Input: part model. Units: mm. Frame: model coordinates. A direction names the side the tool comes from. Coordinates: 2 decimals unless noted, no trailing zeros. Order: outer loops, then holes, each group sorted by start corner. A loop starts at its lowest first (then second) coordinate and runs counter-clockwise, first axis right, second up. Notation, with made-up numbers: (85.5, 15.25) - (93.5, 15.25) arc R13 cw to (93.5, 39.25) - close; hole circle Ø8 at (-19.75, 88.5). An arc over 180 degrees is marked (long way). Use a Markdown table: item, result. Add a question column.
from build123d import *

# Parameters (mm, degrees)
SKETCH_2_R             = 5
EXTRUDE_1_DEPTH        = 0.8
SKETCH_3_W             = 55
SKETCH_3_H             = 2
EXTRUDE_2_DEPTH        = 22
SKETCH_4_R             = 3
EXTRUDE_3_DEPTH        = 2
PATTERN_LINEAR_1_COUNT = 2
PATTERN_LINEAR_1_PITCH = 98
SKETCH_5_R             = 1.6
SKETCH_5_R_2           = 9.5
CUT_EXTRUDE_1_DEPTH    = 2


with BuildPart() as part:
    # 草图2 → 凸台-拉伸1 (new, symmetric)
    with BuildSketch(Plane(origin=(0, 0, 0), x_dir=(1, 0, 0), z_dir=(0, 1, 0))):
        Polygon((-127.5, 75), (-127.5, -75), (-93.5, -75), (-93.5, -48), (-11, -48), (-11, -75), (11, -75), (11, -48), (93.5, -48), (93.5, -75), (127.5, -75), (127.5, 75), (93.5, 75), (93.5, 48), (11, 48), (11, 75), (-11, 75), (-11, 48), (-93.5, 48), (-93.5, 75), align=None)
        with Locations(Location((0, 0, 0), (0, 0, 270))):
            Circle(SKETCH_2_R, mode=Mode.SUBTRACT)
    extrude(amount=EXTRUDE_1_DEPTH, both=True)

    # 草图3 → 凸台-拉伸2 (add)
    with BuildSketch(Plane(origin=(0, 0.8, 0), x_dir=(1, 0, 0), z_dir=(0, 1, 0))):
        with Locations((-44, -47)):
            Rectangle(SKETCH_3_W, SKETCH_3_H)
        with Locations((44, -47)):
            Rectangle(SKETCH_3_W, SKETCH_3_H)
        with Locations((44, 47)):
            Rectangle(SKETCH_3_W, SKETCH_3_H)
        with Locations((-44, 47)):
            Rectangle(SKETCH_3_W, SKETCH_3_H)
    extrude(amount=EXTRUDE_2_DEPTH)

    # 草图4 → 凸台-拉伸3 (add)
    with BuildSketch(Plane.XY.offset(48)):
        with Locations((55.5, 11.8)):
            Circle(SKETCH_4_R)
        with Locations(Location((-55.5, 11.8, 0), (0, 0, 180))):
            Circle(SKETCH_4_R)
    extrude_3 = extrude(amount=EXTRUDE_3_DEPTH)

    # 阵列(线性)1: 凸台-拉伸3 ×2
    with Locations(*[(0, 0, -i * PATTERN_LINEAR_1_PITCH) for i in range(1, PATTERN_LINEAR_1_COUNT)]):
        add(extrude_3)

    # 草图5 → 切除-拉伸1 (cut)
    with BuildSketch(Plane.XZ.offset(0.8)):
        with Locations(Location((-55.5, 0, 0), (0, 0, 270))):
            Circle(SKETCH_5_R)
        with Locations(Location((0, 56.5, 0), (0, 0, 270))):
            Circle(SKETCH_5_R)
        with Locations(Location((7, 70, 0), (0, 0, 270))):
            Circle(SKETCH_5_R)
        with Locations(Location((-7, 70, 0), (0, 0, 270))):
            Circle(SKETCH_5_R)
        with Locations(Location((99, 50, 0), (0, 0, 270))):
            Circle(SKETCH_5_R)
        with Locations(Location((-81.5, -42.5, 0), (0, 0, 270))):
            Circle(SKETCH_5_R)
        with Locations(Location((-50.5, -42.5, 0), (0, 0, 270))):
            Circle(SKETCH_5_R)
        with Locations(Location((-99, -50, 0), (0, 0, 270))):
            Circle(SKETCH_5_R)
        with Locations(Location((-97, 0, 0), (0, 0, 270))):
            Circle(SKETCH_5_R_2)
        with Locations(Location((-121.5, -7, 0), (0, 0, 270))):
            Circle(SKETCH_5_R)
        with Locations(Location((55.5, 0, 0), (0, 0, 90))):
            Circle(SKETCH_5_R)
        with Locations(Location((81.5, -42.5, 0), (0, 0, 90))):
            Circle(SKETCH_5_R)
        with Locations(Location((50.5, -42.5, 0), (0, 0, 90))):
            Circle(SKETCH_5_R)
        with Locations(Location((99, -50, 0), (0, 0, 90))):
            Circle(SKETCH_5_R)
        with Locations(Location((121.5, -7, 0), (0, 0, 90))):
            Circle(SKETCH_5_R)
        with Locations(Location((97, 0, 0), (0, 0, 270))):
            Circle(SKETCH_5_R_2)
        with Locations(Location((7, -70, 0), (0, 0, 90))):
            Circle(SKETCH_5_R)
        with Locations(Location((-7, -70, 0), (0, 0, 90))):
            Circle(SKETCH_5_R)
        with Locations(Location((0, -56.5, 0), (0, 0, 90))):
            Circle(SKETCH_5_R)
        with Locations(Location((50.5, 42.5, 0), (0, 0, 270))):
            Circle(SKETCH_5_R)
        with Locations(Location((81.5, 42.5, 0), (0, 0, 270))):
            Circle(SKETCH_5_R)
        with Locations(Location((121.5, 7, 0), (0, 0, 270))):
            Circle(SKETCH_5_R)
        with Locations(Location((-50.5, 42.5, 0), (0, 0, 90))):
            Circle(SKETCH_5_R)
        with Locations(Location((-121.5, 7, 0), (0, 0, 90))):
            Circle(SKETCH_5_R)
        with Locations(Location((-81.5, 42.5, 0), (0, 0, 90))):
            Circle(SKETCH_5_R)
        with Locations(Location((-99, 50, 0), (0, 0, 90))):
            Circle(SKETCH_5_R)
        with Locations(Location((-79.5, 19, 0), (0, 0, 270))):
            Circle(SKETCH_5_R)
        with Locations(Location((-41.5, 19, 0), (0, 0, 270))):
            Circle(SKETCH_5_R)
        with Locations(Location((-41.5, -19, 0), (0, 0, 90))):
            Circle(SKETCH_5_R)
        with Locations(Location((-79.5, -19, 0), (0, 0, 270))):
            Circle(SKETCH_5_R)
        with Locations(Location((41.5, 19, 0), (0, 0, 90))):
            Circle(SKETCH_5_R)
        with Locations(Location((79.5, 19, 0), (0, 0, 90))):
            Circle(SKETCH_5_R)
        with Locations(Location((41.5, -19, 0), (0, 0, 270))):
            Circle(SKETCH_5_R)
        with Locations(Location((79.5, -19, 0), (0, 0, 270))):
            Circle(SKETCH_5_R)
    extrude(amount=-CUT_EXTRUDE_1_DEPTH, mode=Mode.SUBTRACT)


solid = part.part
1) Cut plane A-A (y = 4.5). Return the cut outline in (x, z).
2) Reachability of faces 1 (the flat face through (44, 12, 46)), 2 (the cylindrical face through (52.5, 11.9, -49)), 3 (the cylindrical face through (52.5, 11.9, 49)) from +Z, -Z, +X, -X, +Y, -Y: full face, straight path, thin tool, end or side. Return the list, or none.
3) Pull-direction query (X, two-part tool) for faces 4 (the cylindrical face through (-4.88, -0.01, -1.08)), 5 (the flat face through (55, 12, -50)); classes: pulls with the +X half, pulls with the -X half, needs draft (parallel to the pull), parting line crosses it, or undercut.
4) Cut plane B-B (x = 46). Return the cut outline in (y, z), and give its area (3 significant figures).
5) Material intervals for L1, parallel to X at y = 0.35, z = -70; L2, parallel to Z at x = 79.5, y = -0.2; L3, parallel to Z at x = -54.5, y = 15.5, sorted ascending.
6) Cut plane C-C (x = 104). Return the cut outline in (y, z).
7) Contact query for flat-ended pins moving along their axis: P1, Ø2, axis at y = 13.5, z = 47.5, coming from the -X side; P2, Ø2, axis at y = 11.5, z = 47.5, coming from the +X side; P3, Ø10, axis at x = -50, y = 10.5, coming from the -Z side. Output: stop coordinate, or through.
Computed:
| question | item | result |
|---|---|---|
| 1 | outline | (-71.5, -48) - (-16.5, -48) - (-16.5, -46) - (-71.5, -46) - close; (-71.5, 46) - (-16.5, 46) - (-16.5, 48) - (-71.5, 48) - close; (16.5, -48) - (71.5, -48) - (71.5, -46) - (16.5, -46) - close; (16.5, 46) - (71.5, 46) - (71.5, 48) - (16.5, 48) - close |
| 2 | face 1 | +X, -X, +Y |
| 2 | face 2 | -Z |
| 2 | face 3 | +Z |
| 3 | face 4 | undercut |
| 3 | face 5 | needs draft |
| 4 | outline | (-0.8, -48) - (22.8, -48) - (22.8, -46) - (0.8, -46) - (0.8, 46) - (22.8, 46) - (22.8, 48) - (-0.8, 48) - close |
| 4 | area | 242 mm2 |
| 5 | L1 | x = -127.5 to -93.5, -11 to -8.6, -5.4 to 5.4, 8.6 to 11, 93.5 to 127.5 |
| 5 | L2 | z = -48 to -20.6, -17.4 to 17.4, 20.6 to 48 |
| 5 | L3 | z = -48 to -46, 46 to 48 |
| 6 | outline | (-0.8, -75) - (0.8, -75) - (0.8, -6.42) - (-0.8, -6.42) - close; (-0.8, 6.42) - (0.8, 6.42) - (0.8, 75) - (-0.8, 75) - close |
| 7 | P1 | stops at x = -71.5 |
| 7 | P2 | stops at x = 71.5 |
| 7 | P3 | stops at z = -50 |
